from build123d import *

# Parameters (mm, degrees)
SKETCH_W     = 16
SKETCH_H     = 50
PAD_DEPTH    = 5
PAD001_DEPTH = 16
SKETCH002_W  = 10
SKETCH002_H  = 50
PAD002_DEPTH = 7
SKETCH003_W  = 10
SKETCH003_H  = 50
PAD003_DEPTH = 7
SKETCH004_R  = 2.625
POCKET_DEPTH = 7


with BuildPart() as part:
    # Sketch → Pad (new body)
    with BuildSketch(Plane.XY):
        Rectangle(SKETCH_W, SKETCH_H)
    extrude(amount=PAD_DEPTH)

    # Sketch001 (on Face3 of Pad) → Pad001 (join)
    with BuildSketch(Plane.YZ.offset(8)):
        Polygon((-23.75, 5), (-23.5, 6), (-21.5, 6), (-21.25, 5), align=None)
        Polygon((-18.75, 5), (-18.5, 6), (-16.5, 6), (-16.25, 5), align=None)
        Polygon((-13.75, 5), (-13.5, 6), (-11.5, 6), (-11.25, 5), align=None)
        Polygon((-8.75, 5), (-8.5, 6), (-6.5, 6), (-6.25, 5), align=None)
        Polygon((-3.75, 5), (-3.5, 6), (-1.5, 6), (-1.25, 5), align=None)
        Polygon((1.25, 5), (1.5, 6), (3.5, 6), (3.75, 5), align=None)
        Polygon((6.25, 5), (6.5, 6), (8.5, 6), (8.75, 5), align=None)
        Polygon((11.25, 5), (11.5, 6), (13.5, 6), (13.75, 5), align=None)
        Polygon((16.25, 5), (16.5, 6), (18.5, 6), (18.75, 5), align=None)
        Polygon((21.25, 5), (21.5, 6), (23.5, 6), (23.75, 5), align=None)
    extrude(amount=-PAD001_DEPTH)

    # Sketch002 (on Face4 of Pad001) → Pad002 (join)
    with BuildSketch(Plane(origin=(0, 0, 0), x_dir=(1, 0, 0), z_dir=(0, 0, -1))):
        with Locations((13, 0)):
            Rectangle(SKETCH002_W, SKETCH002_H)
    extrude(amount=-PAD002_DEPTH)

    # Sketch003 (on Face4 of Pad002) → Pad003 (join)
    with BuildSketch(Plane(origin=(0, 0, 0), x_dir=(1, 0, 0), z_dir=(0, 0, -1))):
        with Locations((-13, 0)):
            Rectangle(SKETCH003_W, SKETCH003_H)
    extrude(amount=-PAD003_DEPTH)

    # Sketch004 (on Face12 of Pad003) → Pocket (cut)
    with BuildSketch(Plane(origin=(0, 0, 0), x_dir=(1, 0, 0), z_dir=(0, 0, -1))):
        with Locations((-12.5, 20)):
            Circle(SKETCH004_R)
        with Locations((-12.5, -20)):
            Circle(SKETCH004_R)
        with Locations((12.5, -20)):
            Circle(SKETCH004_R)
        with Locations((12.5, 20)):
            Circle(SKETCH004_R)
    extrude(amount=-POCKET_DEPTH, mode=Mode.SUBTRACT)


solid = part.part
The listing builds one solid part. Answer for the finished solid, in the listing's coordinates (mm). A direction names the side the tool comes from. Give positions to 0.01 mm unless a question says otherwise; leave off trailing zeros. Write each loop counter-clockwise with the first axis right and the second up, starting at its lowest first coordinate (ties: lowest second). Pieces come first, ordered by that corner, then holes.
1) Given P1, Ø1.6, axis at x = 0.5, y = 7.5, coming from the +Z side; P2, Ø0.8, axis at x = -1, y = -9.5, coming from the +Z side, each flat-ended and moving along its own axis, determine where each tip first touches the part or whether it passes through.
2) Section B-B (y = -20) is taken. Write down the section's boundary in (x, z) (3 decimals), and give its area (4 significant figures).
3) Section C-C (x = -12.5) is taken. Write down the section's boundary in (y, z) (3 decimals).
4) Section D-D (y = 7.5) is taken. Write down the section's boundary in (x, z).
5) Section A-A (z = 4) is taken. Write down the section's boundary in (x, y) (3 decimals), and give its area (3 significant figures).
6) Find the intervals of material crossed by L1, parallel to X at y = -20, z = 5.25 (3 decimals); L2, parallel to Y at x = -12.5, z = 5.5 (3 decimals); L3, parallel to X at y = 20, z = 2 (3 decimals), in increasing order.
7) A tool of negligible diameter and unlimited length cuts with its end or side. For faces 3 (the face through (0, 2, 6)), 4 (the face through (0.112, 16.373, 5.493)), 5 (the face through (0.112, -23.627, 5.493)), from which of +Z, -Z, +X, -X, +Y, -Y can it reach the whole face along a straight path? Write none if from no direction.
8) For a pull along X with two mould halves and no side action, classify faces 1 (the face through (0, 25, 3)), 2 (the face through (0, 22, 6)) as pulls with the +X half, pulls with the -X half, needs draft (parallel to the pull), parting line crosses it, or undercut.
Response:
1. P1: stops at z = 6
1. P2: stops at z = 5
2. outline: (-18, 0) - (-15.125, 0) - (-15.125, 7) - (-18, 7) - close; (-9.875, 0) - (9.875, 0) - (9.875, 7) - (8, 7) - (8, 5) - (-8, 5) - (-8, 7) - (-9.875, 7) - close; (15.125, 0) - (18, 0) - (18, 7) - (15.125, 7) - close
2. area: 146.5 mm2
3. outline: (-25, 0) - (-22.625, 0) - (-22.625, 7) - (-25, 7) - close; (-17.375, 0) - (17.375, 0) - (17.375, 7) - (-17.375, 7) - close; (22.625, 0) - (25, 0) - (25, 7) - (22.625, 7) - close
4. outline: (-18, 0) - (18, 0) - (18, 7) - (8, 7) - (8, 6) - (-8, 6) - (-8, 7) - (-18, 7) - close
5. outline: (-18, -25) - (18, -25) - (18, 25) - (-18, 25) - close; hole circle Ø5.25 at (-12.5, -20); hole circle Ø5.25 at (-12.5, 20); hole circle Ø5.25 at (12.5, -20); hole circle Ø5.25 at (12.5, 20)
5. area: 1,710 mm2
6. L1: x = -18 to -15.125, -9.875 to -8, 8 to 9.875, 15.125 to 18
6. L2: y = -25 to -22.625, -17.375 to 17.375, 22.625 to 25
6. L3: x = -18 to -15.125, -9.875 to 9.875, 15.125 to 18
7. face 3: +Z, +Y, -Y
7. face 4: +Z
7. face 5: +Z, -Y
8. face 1: needs draft
8. face 2: undercut
